Can you work these out from the model? Positions are in its coordinate system, mm. Coordinates: 2 decimals unless noted, no trailing zeros. Write each loop counter-clockwise with the first axis right and the second up, starting at its lowest first coordinate (ties: lowest second). Pieces come first, ordered by that corner, then holes. Notation, with made-up numbers: (0, -2.5) - (29, -2.5) arc R12 cw to (29, 17.5) - close; hole circle Ø6 at (-31.5, -7.75). An arc over 180 degrees is marked (long way). Use one line per item in the form item = value. Start each with the question number.
(1) For pin 1 Ø4.5 at (x, z) = (-39.5, -35.1) entering from -Y; pin 2 Ø2 at (x, z) = (-79.5, -75.1) entering from -Y, each with a flat end and sliding along its axis, tell me the tip position at first contact or that it passes through.
(2) If we section it at A-A on z = -55.1: Please give me the cut outline in (x, y).
(3) Thinking about a two-plate mould opening in Z: for faces 1 (the face through (-78.253, 1.268, -34.583)), 2 (the face through (-59, 1, 0)), 3 (the face through (-59, 0, -79)), which applies, pulls with the +Z half, pulls with the -Z half, needs draft (parallel to the pull), parting line crosses it, or undercut?
(4) If we section it at B-B on x = -59.5: Please give me the cut outline in (y, z), then the cut area to 4 significant figures.
(5) If we section it at C-C on z = -105.95: Please give me the cut outline in (x, y) (3 decimals), then the cut area to 3 significant figures.
(6) If we section it at D-D on y = 1.45: Give the number of separate pieces and of enclosed holes in the cut face, then the cut area to 3 significant figures.
(7) If I drill on probe 1 along X at (y, z) = (1.3, -105.95) (3 decimals); probe 2 along Z at (x, y) = (-60.5, 0.55); probe 3 along Z at (x, y) = (-66, 1.85), over which ranges is the centre line in solid material (lowest first)? Write a range as from..to.
Autodesk Inventor part; units mm, degrees
ref_plane "Work Plane1" through (-59.5, 0, 0) normal (1, 0, 0) x (0, 0, -1)
ref_plane "YZ Plane" through (0, 0, 0) normal (1, 0, 0) x (0, 1, 0)
ref_plane "XZ Plane" through (0, 0, 0) normal (0, 1, 0) x (-1, 0, 0)
sketch "Sketch1" plane through (0, 0, 0) normal (0, 1, 0) x (-1, 0, 0)
  line L0 (0, 0) -> (119, 0)
  line L1 (119, 0) -> (119, -110.2)
  line L2 (119, -110.2) -> (0, -110.2)
  line L3 (0, -110.2) -> (0, 0)
  dimension "d0" = 119
  dimension "d1" = 110.2
extrude "Extrusion1" add sketch "Sketch1" along normal blind 2.5
sketch "Sketch2" plane through (0, 2.5, 0) normal (0, 1, 0) x (1, 0, 0)
  line L0 (-119, 0) -> (0, 0)
  line L1 (0, 0) -> (0, 110.2)
  line L2 (0, 110.2) -> (-119, 110.2)
  line L3 (-119, 110.2) -> (-119, 0)
  circle A0 centre (-114.875, 4.375) radius 1.55
  circle A1 centre (-11.5301, 10.067) radius 1.55
  circle A2 centre (-11.5301, 99.7072) radius 1.55
  circle A3 centre (-114.875, 105.95) radius 1.55
  dimension "d4" = 3.1
  dimension "d5" = 3.1
  dimension "d6" = 3.1
  dimension "d7" = 3.1
  dimension "d8" = 4.375
  dimension "d9" = 4.125
  dimension "d10" = 4.25
  dimension "d11" = 4.125
extrude "Extrusion2" cut sketch "Sketch2" against normal through all contours A0 | A3
ref_plane "Work Plane1" through (-59.5, 0, 0) normal (1, 0, 0) x (0, 0, -1)
mirror "Mirror1" about plane through (-59.5, 0, 0) normal (1, 0, 0) of "Extrusion2"
sketch "Sketch3" plane through (0, 2.5, 0) normal (0, 1, 0) x (1, 0, 0)
  circle A0 centre (-4.125, 4.375) radius 1.55
  circle A1 centre (-4.125, 105.95) radius 1.55
  circle A2 centre (-114.875, 4.375) radius 1.55
  circle A3 centre (-114.875, 105.95) radius 1.55
  line L0 (-119, 0) -> (0, 0)
  line L1 (0, 0) -> (0, 110.2)
  line L2 (0, 110.2) -> (-119, 110.2)
  line L3 (-119, 110.2) -> (-119, 0)
  circle A4 centre (-59.5, 55.1) radius 20
  circle A5 centre (-39.5, 75.1) radius 1.35
  circle A6 centre (-39.5, 35.1) radius 1.35
  circle A7 centre (-79.5, 35.1) radius 1.35
  circle A8 centre (-79.5, 75.1) radius 1.35
  dimension "d26" = 2.7
  dimension "d27" = 2.7
extrude "Extrusion3" cut sketch "Sketch3" against normal through all contours A4 | A5 | A6 | A7 | A8
properties part number "Base Cover Left"
Reported:
q1.pin_1 = 0
q1.pin_2 = through
q2.outline = (-119, 0) - (-79.5, 0) - (-79.5, 2.5) - (-119, 2.5) - close; (-39.5, 0) - (0, 0) - (0, 2.5) - (-39.5, 2.5) - close
q3.face_1 = undercut
q3.face_2 = pulls with the +Z half
q3.face_3 = needs draft
q4.outline = (0, -110.2) - (2.5, -110.2) - (2.5, -75.1) - (0, -75.1) - close; (0, -35.1) - (2.5, -35.1) - (2.5, 0) - (0, 0) - close
q4.area = 175.5 mm2
q5.outline = (-119, 0) - (-116.425, 0) - (-116.425, 2.5) - (-119, 2.5) - close; (-113.325, 0) - (-5.675, 0) - (-5.675, 2.5) - (-113.325, 2.5) - close; (-2.575, 0) - (0, 0) - (0, 2.5) - (-2.575, 2.5) - close
q5.area = 282 mm2
q6.separate_pieces = 1
q6.enclosed_holes = 9
q6.area = 11,800 mm2
q7.probe_1 = -119..-116.425, -113.325..-5.675, -2.575..0
q7.probe_2 = -110.2..-75.07, -35.13..0
q7.probe_3 = -110.2..-74.01, -36.19..0
